Source: CAD feature listing. Evaluate the final solid. Frame: model axes, mm. Round coordinates to 2 decimals unless told otherwise and drop trailing zeros. Loops run counter-clockwise (first coordinate to the right, second up) from the corner with the lowest first, then second, coordinate; pieces in that order, holes last. Notation, with made-up numbers: (23, -37) - (82, -37) arc R25 cw to (82, -20) - close; hole circle Ø7 at (-14.5, 11.25). An arc over 180 degrees is marked (long way). Write item = value, one per line. Start each with the question number.
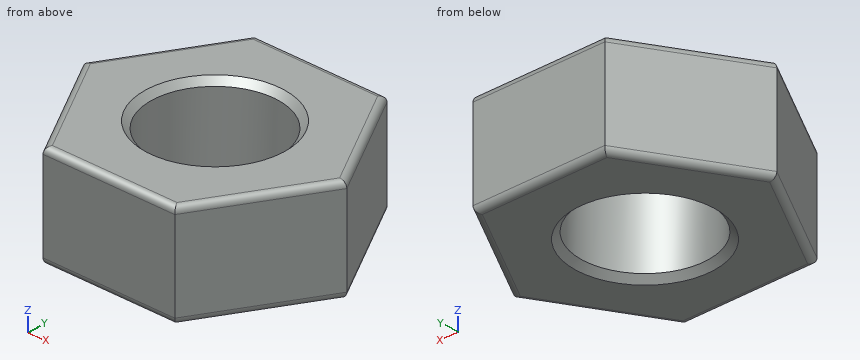
from build123d import *

# Parameters (mm, degrees)
F2_R     = 1.5
F3_DEPTH = 2.4
F4_R     = 0.15
F5_SIZE  = 0.15


with BuildPart() as f3:
    # F2 (on Top) → F3 (new body)
    with BuildSketch(Plane.XY):
        Polygon((1.5877132403, 2.75), (-1.5877132403, 2.75), (-3.1754264805, 0), (-1.5877132403, -2.75), (1.5877132403, -2.75), (3.1754264805, 0), align=None)
        Circle(F2_R, mode=Mode.SUBTRACT)
    extrude(amount=F3_DEPTH)

    # F4
    f4_edges = [f3.edges().sort_by_distance(p)[0] for p in [
        (2.38157, -1.375, 2.4),
        (2.38157, 1.375, 2.4),
        (0, 2.75, 2.4),
        (-2.38157, 1.375, 2.4),
        (-2.38157, -1.375, 2.4),
        (0, -2.75, 2.4),
        (0, -2.75, 0),
        (2.38157, -1.375, 0),
        (-2.38157, -1.375, 0),
        (-2.38157, 1.375, 0),
        (0, 2.75, 0),
        (2.38157, 1.375, 0),
    ]]
    fillet(f4_edges, radius=F4_R)

    # F5
    f5_edges = [f3.edges().sort_by_distance(p)[0] for p in [
        (-1.5, 0, 2.4),
        (-1.5, 0, 0),
    ]]
    chamfer(f5_edges, length=F5_SIZE)


solid = f3.part
(1) Cut plane A-A (x = 0). Output: boundary loops of the cut face in (y, z).
(2) Cut plane B-B (z = 0.55). Output: boundary loops of the cut face in (x, y).
(3) Pin query (flat end, axial travel): P1, Ø1, axis at y = -1.5, z = 1.5, coming from the +X side. Return the tip coordinate at first contact, or that it passes through.
(4) Material intervals for line 1 along Y through (x, z) = (0, 1.45); line 2 along Y through (x, z) = (-0.75, 1.45); line 3 along Z through (x, y) = (1.5, -0.4), sorted ascending. Write a range as from..to.
Solution:
q1.outline = (-2.75, 0.15) arc R0.15 ccw to (-2.6, 0) - (-1.65, 0) - (-1.5, 0.15) - (-1.5, 2.25) - (-1.65, 2.4) - (-2.6, 2.4) arc R0.15 ccw to (-2.75, 2.25) - close; (1.5, 0.15) - (1.65, 0) - (2.6, 0) arc R0.15 ccw to (2.75, 0.15) - (2.75, 2.25) arc R0.15 ccw to (2.6, 2.4) - (1.65, 2.4) - (1.5, 2.25) - close
q2.outline = (-3.18, 0) - (-1.59, -2.75) - (1.59, -2.75) - (3.18, 0) - (1.59, 2.75) - (-1.59, 2.75) - close; hole circle Ø3 at (0, 0)
q3.P1 = 2.6
q4.line_1 = -2.75..-1.5, 1.5..2.75
q4.line_2 = -2.75..-1.3, 1.3..2.75
q4.line_3 = 0.1..2.3
